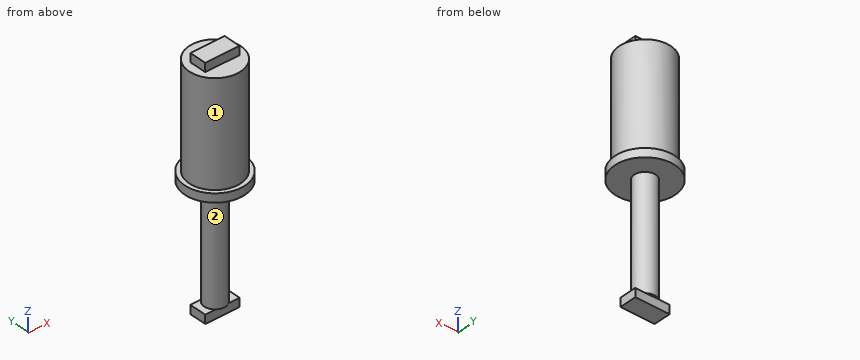
from build123d import *

# Parameters (mm, degrees)
SKETCH1_R           = 12.5
BOSS_EXTRUDE1_DEPTH = 130
SKETCH2_R           = 35
BOSS_EXTRUDE2_DEPTH = 10
SKETCH3_R           = 30
BOSS_EXTRUDE3_DEPTH = 120
SKETCH4_W           = 40
SKETCH4_H           = 20
BOSS_EXTRUDE4_DEPTH = 10
SCHIZZO1_W          = 40
SCHIZZO1_H          = 20
BOSS_EXTRUDE5_DEPTH = 10


with BuildPart() as part:
    # Sketch1 → Boss-Extrude1 (new body)
    with BuildSketch(Plane.XY):
        Circle(SKETCH1_R)
    extrude(amount=BOSS_EXTRUDE1_DEPTH)

    # Sketch2 → Boss-Extrude2 (add)
    with BuildSketch(Plane.XY.offset(130)):
        Circle(SKETCH2_R)
    extrude(amount=BOSS_EXTRUDE2_DEPTH)

    # Sketch3 → Boss-Extrude3 (add)
    with BuildSketch(Plane.XY.offset(140)):
        Circle(SKETCH3_R)
    extrude(amount=BOSS_EXTRUDE3_DEPTH)

    # Sketch4 → Boss-Extrude4 (add)
    with BuildSketch(Plane(origin=(0, 0, 0), x_dir=(-1, 0, 0), z_dir=(0, 0, -1))):
        Rectangle(SKETCH4_W, SKETCH4_H)
    extrude(amount=BOSS_EXTRUDE4_DEPTH)

    # Schizzo1 → Boss-Extrude5 (add)
    with BuildSketch(Plane.XY.offset(260)):
        Rectangle(SCHIZZO1_W, SCHIZZO1_H)
    extrude(amount=BOSS_EXTRUDE5_DEPTH)


solid = part.part
Read the model definition and answer for the solid it produces. Units are mm, in the model's axes. Face numbers are marked on the shaded views. Give positions to 0.01 mm unless a question says otherwise; leave off trailing zeros. Write each loop counter-clockwise with the first axis right and the second up, starting at its lowest first coordinate (ties: lowest second). Pieces come first, ordered by that corner, then holes. Notation, with made-up numbers: M 74.25,13.25 L 83.25,13.25 A14 cw 83.25,28.25 Z; hole C -35.5,3.25 d3. An arc over 180 degrees is marked long. One line per item, written item: value. Start each with the question number.
(1) Find section D-D (y = 17.5). Determine the outline of the cut face in (x, z).
(2) Find the intervals of material crossed by line 1 (Z direction, x = -17, y = 5); line 2 (Z direction, x = -10, y = -15.5); line 3 (Z direction, x = -20, y = 28), in increasing order.
(3) Find section B-B (y = 0). Determine the outline of the cut face in (x, z).
(4) Flat-ended cylindrical pins translate along their axes: pin 1 Ø1 at (x, z) = (4.5, 54) entering from -Y; pin 2 Ø12 at (x, y) = (-17, -20) entering from -Z; pin 3 Ø8 at (y, z) = (-2.5, 265.5) entering from -X. Find the tip coordinate at first contact, or state that the pin passes through.
(5) Find section A-A (x = 0). Determine the outline of the cut face in (y, z).
(6) Determine the mould class of the marked faces 1 and 2 for opening direction Z: pulls with the +Z half, pulls with the -Z half, needs draft (parallel to the pull), parting line crosses it, or undercut.
(7) Find section C-C (z = 133.5). Determine the outline of the cut face in (x, y).
Results below:
1. outline: M -30.31,130 L 30.31,130 L 30.31,140 L 24.37,140 L 24.37,260 L -24.37,260 L -24.37,140 L -30.31,140 Z
2. line 1: z = -10 to 0, 130 to 270
2. line 2: z = 130 to 260
2. line 3: z = 130 to 140
3. outline: M -35,130 L -12.5,130 L -12.5,0 L -20,0 L -20,-10 L 20,-10 L 20,0 L 12.5,0 L 12.5,130 L 35,130 L 35,140 L 30,140 L 30,260 L 20,260 L 20,270 L -20,270 L -20,260 L -30,260 L -30,140 L -35,140 Z
4. pin 1: stops at y = -11.84
4. pin 2: stops at z = 130
4. pin 3: stops at x = -20
5. outline: M -35,130 L -12.5,130 L -12.5,0 L -10,0 L -10,-10 L 10,-10 L 10,0 L 12.5,0 L 12.5,130 L 35,130 L 35,140 L 30,140 L 30,260 L 10,260 L 10,270 L -10,270 L -10,260 L -30,260 L -30,140 L -35,140 Z
6. face 1: needs draft
6. face 2: undercut
7. outline: C 0,0 d70
